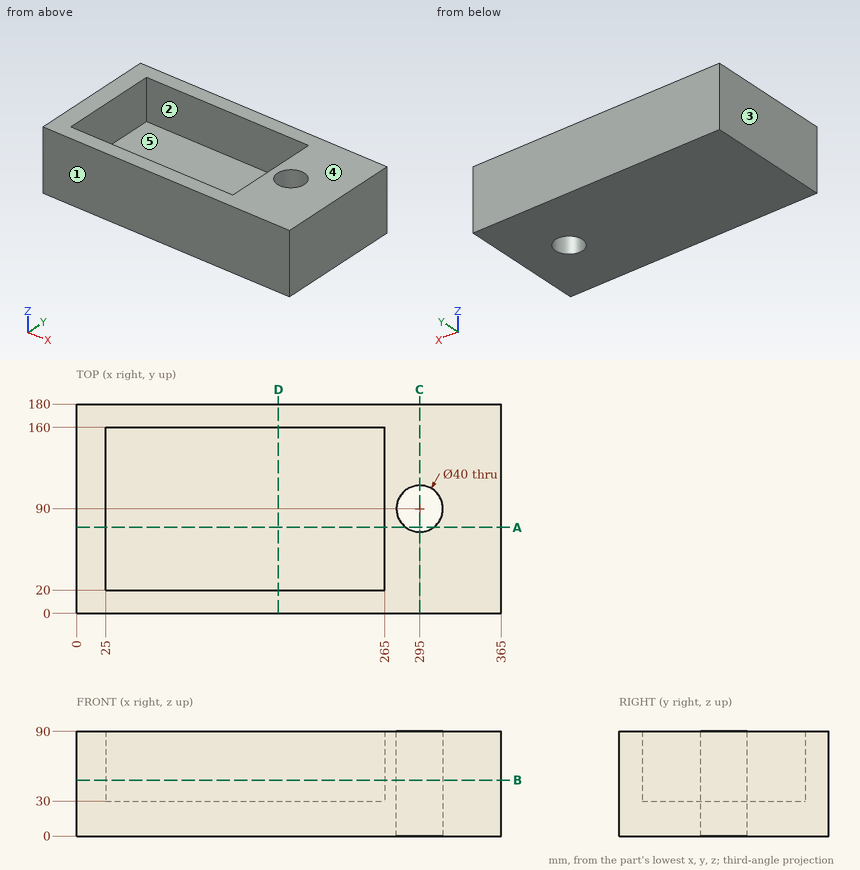
Could you check a few things on this drawing? It's one solid part, dimensions in mm from its lowest x, y, z. A direction names the side the tool comes from. Give positions to 0.01 mm unless a question says otherwise; leave off trailing zeros. Order: outer loops, then holes, each group sorted by start corner. A loop starts at its lowest first (then second) coordinate and runs counter-clockwise, first axis right, second up. Notation, with made-up numbers: M 36,79 L 69,79 A12 cw 69,91 Z; hole C 81.5,1 d10. An arc over 180 degrees is marked long. Use one line per item in the form item = value. Start each with the question number.
Item 1: If we section it at C-C (x = 295): Write out the boundary of the cut face in (y, z), then the cut area to 3 significant figures.
Item 2: If we section it at A-A (y = 74): Write out the boundary of the cut face in (x, z), then the cut area to 3 significant figures.
Item 3: Will this pin go through, and if not, where does the flat tip stop? pin 1 Ø10 at (x, y) = (67.5, 111) entering from +Z.
Item 4: If I drill on line 1 along Y through (x, z) = (295, 46); line 2 along Y through (x, z) = (199, 48); line 3 along X through (y, z) = (79, 78), over which ranges is the centre line in solid material (lowest first)?
Item 5: We'd pull the mould along X, two halves only. Please class the marked faces 3, 4 and 5: +X half, -X half, draft (parallel to the pull), parting line (faces both ways), or undercut.
Item 6: For the marked faces 1 and 2, which set-ups out of +Z, -Z, +X, -X, +Y, -Y let a thin tool reach every point of the face, with its end or its side?
Item 7: If we section it at D-D (x = 173.5): Write out the boundary of the cut face in (y, z), then the cut area to 3 significant figures.
Item 8: If we section it at B-B (z = 48): Write out the boundary of the cut face in (x, y), then the cut area to 3 significant figures.
Outcome:
q1.outline = M 0,0 L 70,0 L 70,90 L 0,90 Z; M 110,0 L 180,0 L 180,90 L 110,90 Z
q1.area = 12,600 mm2
q2.outline = M 0,0 L 283,0 L 283,90 L 265,90 L 265,30 L 25,30 L 25,90 L 0,90 Z; M 307,0 L 365,0 L 365,90 L 307,90 Z
q2.area = 16,300 mm2
q3.pin_1 = 30
q4.line_1 = 0 to 70, 110 to 180
q4.line_2 = 0 to 20, 160 to 180
q4.line_3 = 0 to 25, 265 to 278.3, 311.7 to 365
q5.face_3 = -X half
q5.face_4 = draft
q5.face_5 = undercut
q6.face_1 = +Z, -Z, +X, -X, -Y
q6.face_2 = +Z
q7.outline = M 0,0 L 180,0 L 180,90 L 160,90 L 160,30 L 20,30 L 20,90 L 0,90 Z
q7.area = 7,800 mm2
q8.outline = M 0,0 L 365,0 L 365,180 L 0,180 Z; hole M 25,20 L 265,20 L 265,160 L 25,160 Z; hole C 295,90 d40
q8.area = 30,800 mm2
